The figure shows three views and two pictorial views of one solid part (mm, origin at its lowest corner). Answer the questions. A direction names the side the tool comes from. Coordinates: 2 decimals unless noted, no trailing zeros. Order: outer loops, then holes, each group sorted by start corner. A loop starts at its lowest first (then second) coordinate and runs counter-clockwise, first axis right, second up. Notation, with made-up numbers: M 53,88 L 75,88 A13 ccw 75,92 Z; hole C 53.5,33 d2. An arc over 180 degrees is marked long. Answer in a Markdown table with one row per item. Add a question column.
Item 1: Flat-ended cylindrical pins translate along their axes: pin 1 Ø5 at (y, z) = (85, 7.5) entering from -X (3 decimals); pin 2 Ø6 at (x, z) = (11.5, 8) entering from -Y; pin 3 Ø3.5 at (x, z) = (18, 7.5) entering from +Y. Find the tip coordinate at first contact, or state that the pin passes through.
Item 2: The part is cut by section D-D (y = 23). Write down the section's boundary in (x, z) (1 decimal).
Item 3: Which of the six approach directions +Z, -Z, +X, -X, +Y, -Y give full straight-line access (tool end or side, diameter ignored) to the marked faces 1, 2 and 3?
Item 4: The mould has two halves that part along Z. Classify the marked faces 4, 5 and 6: released by +Z, released by -Z, zero draft, split by the parting line, or undercut.
Item 5: The part is cut by section C-C (x = 9.25). Write down the section's boundary in (y, z).
Item 6: Consider line 1 (Z direction, x = 5.75, y = 26.5); line 2 (Y direction, x = 5.75, z = 15.5); line 3 (X direction, y = 79, z = 1.75) (1 decimal). Determine where each line is inside the solid, lowest interval first. Write a range as from..to.
Item 7: The part is cut by section A-A (y = 51). Write down the section's boundary in (x, z) (1 decimal).
Item 8: The part is cut by section B-B (z = 6.5). Write down the section's boundary in (x, y) (1 decimal), then the cut area to 3 significant figures.
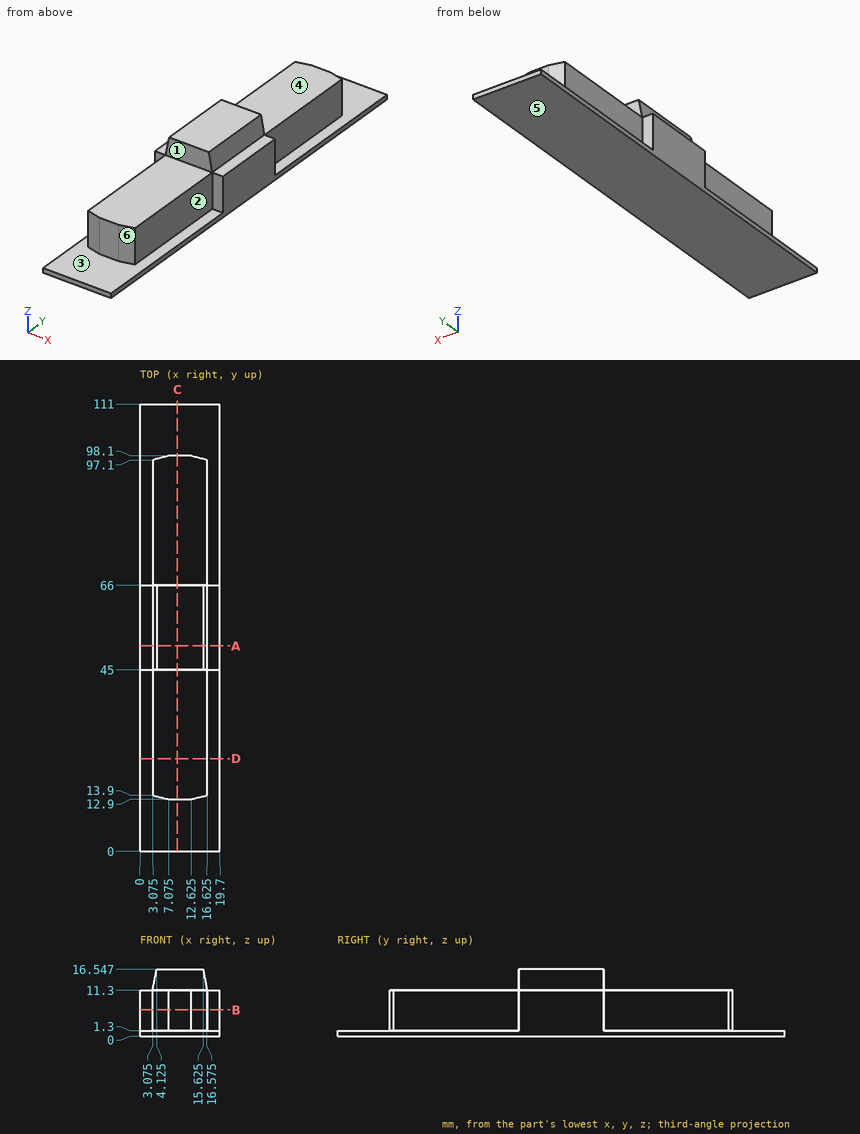
Reply:
| question | item | result |
|---|---|---|
| 1 | pin 1 | stops at x = 3.075 |
| 1 | pin 2 | stops at y = 12.9 |
| 1 | pin 3 | stops at y = 97.19 |
| 2 | outline | M 0,0 L 19.7,0 L 19.7,1.3 L 16.6,1.3 L 16.6,11.3 L 3.1,11.3 L 3.1,1.3 L 0,1.3 Z |
| 3 | face 1 | +Z, +X, -X, -Y |
| 3 | face 2 | +Z, +X, -Y |
| 3 | face 3 | +Z, -Y |
| 4 | face 4 | released by +Z |
| 4 | face 5 | released by -Z |
| 4 | face 6 | zero draft |
| 5 | outline | M 0,0 L 111,0 L 111,1.3 L 98.1,1.3 L 98.1,11.3 L 66,11.3 L 66,16.55 L 45,16.55 L 45,11.3 L 12.9,11.3 L 12.9,1.3 L 0,1.3 Z |
| 6 | line 1 | z = 0..11.3 |
| 6 | line 2 | y = 45..66 |
| 6 | line 3 | x = 3.1..16.6 |
| 7 | outline | M 0,0 L 19.7,0 L 19.7,11.3 L 16.6,11.3 L 15.6,16.5 L 4.1,16.5 L 3.1,11.3 L 0,11.3 Z |
| 8 | outline | M 0,45 L 3.1,45 L 3.1,13.9 L 7.1,12.9 L 12.6,12.9 L 16.6,13.9 L 16.6,45 L 19.7,45 L 19.7,66 L 16.6,66 L 16.6,97.1 L 12.6,98.1 L 7.1,98.1 L 3.1,97.1 L 3.1,66 L 0,66 Z |
| 8 | area | 1,280 mm2 |
